from build123d import *

# Parameters (mm, degrees)
SKIZZE1_W                       = 50
SKIZZE1_H                       = 80
AUFSATZ_LINEAR_AUSTRAGEN1_DEPTH = 25
F_6_0_6_DURCHMESSER_BOHRUNG1_D  = 6


with BuildPart() as part:
    # Skizze1 → Aufsatz-Linear austragen1 (new body, symmetric)
    with BuildSketch(Plane(origin=(0, 0, 0), x_dir=(0, 0, -1), z_dir=(1, 0, 0))):
        with Locations((0, 10)):
            Rectangle(SKIZZE1_W, SKIZZE1_H)
    extrude(amount=AUFSATZ_LINEAR_AUSTRAGEN1_DEPTH, both=True)

    # Skizze2 → Schnitt-Rotation1 (revolve, cut)
    with BuildSketch(Plane(origin=(0, 0, 0), x_dir=(0, 0, -1), z_dir=(1, 0, 0)), mode=Mode.PRIVATE) as schnitt_rotation1_sk:
        Polygon((0, 50), (0, -23.004303095), (5, -20), (5, 40), (10, 40), (10, 45), (11.2, 45), (11.2, 47), (10, 47), (10, 50), align=None)
    revolve(schnitt_rotation1_sk.sketch.rotate(Axis((0, -23.004303095, 0), (0, -1, 0)), 180), axis=Axis((0, -23.004303095, 0), (0, -1, 0)), mode=Mode.SUBTRACT)  # turned: the seam where the file's is

    # Ø6.0 (6) Durchmesser Bohrung1 (through all)
    with Locations(Plane(origin=(25, 0, 0), x_dir=(0, 0, -1), z_dir=(1, 0, 0))):
        with Locations((0, 0)):
            Hole(F_6_0_6_DURCHMESSER_BOHRUNG1_D / 2)


solid = part.part
Work out the finished part from the listing and answer in its coordinate system (mm). A direction names the side the tool comes from. Give positions to 0.01 mm unless a question says otherwise; leave off trailing zeros. Order: outer loops, then holes, each group sorted by start corner. A loop starts at its lowest first (then second) coordinate and runs counter-clockwise, first axis right, second up. Notation, with made-up numbers: (2, 79.25) -> (8, 79.25) arc R12 cw to (8, 95.25) -> close; hole circle Ø4 at (36.25, 29.25). An arc over 180 degrees is marked (long way). Answer as a JSON object with one key per item and string values. Group by question number.
1. Section B-B on y = 21 is taken. Determine the outline of the cut face in (x, z).
2. The mould has two halves that part along Z. Classify faces 4 (the flat face through (-25, 11, 0)), 5 (the flat face through (0, 9, 25)), 6 (the cylindrical face through (14, 0, -3)): released by +Z, released by -Z, zero draft, split by the parting line, or undercut.
3. Flat-ended cylindrical pins translate along their axes: pin 1 Ø10 at (x, z) = (-4, -1) entering from +Y; pin 2 Ø6 at (x, z) = (0, 0) entering from +Y; pin 3 Ø9.5 at (y, z) = (0, 0) entering from +X. Find the tip coordinate at first contact, or state that the pin passes through.
4. Section C-C on z = 9 is taken. Determine the outline of the cut face in (x, y), plus the area to 3 significant figures.
5. Consider line 1 along X through (y, z) = (9.5, 3); line 2 along Y through (x, z) = (12, 0); line 3 along Z through (x, y) = (19, 0). Determine where each line is inside the solid, lowest interval first. Write a range as [from, to].
6. Section A-A on y = 0 is taken. Determine the outline of the cut face in (x, z).
7. A tool of negligible diameter and unlimited length cuts with its end or side. For faces 1 (the cylindrical face through (-0.49, 46.01, -11.19)), 2 (the flat face through (0, 9, -25)), 3 (the cylindrical face through (4.88, 10.42, -1.08)), from which of +Z, -Z, +X, -X, +Y, -Y can it reach the whole face along a straight path? Write none if from no direction.
Result sheet:
{
 "1": {"outline": "(-25, -25) -> (25, -25) -> (25, 25) -> (-25, 25) -> close; hole circle Ø10 at (0, 0)"},
 "2": {"face 4": "zero draft", "face 5": "released by +Z", "face 6": "undercut"},
 "3": {"pin 1": "stops at y = 40", "pin 2": "stops at y = -21.2", "pin 3": "stops at x = 25"},
 "4": {"outline": "(-25, -30) -> (25, -30) -> (25, 50) -> (4.36, 50) -> (4.36, 47) -> (6.67, 47) -> (6.67, 45) -> (4.36, 45) -> (4.36, 40) -> (-4.36, 40) -> (-4.36, 45) -> (-6.67, 45) -> (-6.67, 47) -> (-4.36, 47) -> (-4.36, 50) -> (-25, 50) -> close", "area": "3,900 mm^2"},
 "5": {"line 1": "x = [-25, -4], [4, 25]", "line 2": "y = [-30, -3], [3, 50]", "line 3": "z = [-25, -3], [3, 25]"},
 "6": {"outline": "(-25, -25) -> (25, -25) -> (25, -3) -> (4, -3) arc R5 cw to (-4, -3) -> (-25, -3) -> close; (-25, 3) -> (-4, 3) arc R5 cw to (4, 3) -> (25, 3) -> (25, 25) -> (-25, 25) -> close"},
 "7": {"face 1": "none", "face 2": "-Z, +X, -X, +Y, -Y", "face 3": "+Y"}
}
